Read the model definition and answer for the solid it produces. Units are mm, in the model's axes. Give positions to 0.01 mm unless a question says otherwise; leave off trailing zeros. Order: outer loops, then holes, each group sorted by start corner. A loop starts at its lowest first (then second) coordinate and runs counter-clockwise, first axis right, second up. Notation, with made-up numbers: (-35, 66) - (-27, 66) arc R23 ccw to (-27, 90) - close; hole circle Ø9 at (-23, -22.5). An arc over 180 degrees is marked (long way). Write item = value, one per line.
```python
from build123d import *

# Parameters (mm, degrees)
SKETCH1_R           = 46.575911091
SKETCH1_R_2         = 1.5875
BOSS_EXTRUDE1_DEPTH = 3.175


with BuildPart() as part:
    # Sketch1 → Boss-Extrude1 (new body)
    with BuildSketch(Plane(origin=(0, 0, 0), x_dir=(1, 0, 0), z_dir=(0, 1, 0))):
        with Locations(Location((-1e-09, -8.701819906, 0), (0, 0, 270))):
            Circle(SKETCH1_R)
        with Locations(Location((-21.062340002, 28.785905516, 0), (0, 0, 270))):
            Circle(SKETCH1_R_2, mode=Mode.SUBTRACT)
        with Locations(Location((20.847659998, 28.785905516, 0), (0, 0, 270))):
            Circle(SKETCH1_R_2, mode=Mode.SUBTRACT)
        with BuildLine():
            Line((17.640592508, -35.322668494), (1.122532008, -18.804607993))
            ThreePointArc((1.122532008, -18.804607993), (-8e-09, -18.339640008), (-1.122532023, -18.804607993))
            Line((-1.122532023, -18.804607993), (-17.640592542, -35.322668513))
            ThreePointArc((-17.640592542, -35.322668513), (-18.093334403, -36.641843516), (-17.330191572, -37.809238437))
            ThreePointArc((-17.330191572, -37.809238437), (-1.3e-08, -42.577730996), (17.330191539, -37.809238417))
            ThreePointArc((17.330191539, -37.809238417), (18.09333437, -36.641843496), (17.640592508, -35.322668494))
        make_face(mode=Mode.SUBTRACT)
        Polygon((-18.9752812, 8.136160364), (-16.837980243, 10.27346132), (-7.965487196, 1.400968273), (-10.102788153, -0.736332684), align=None, mode=Mode.SUBTRACT)
        with BuildLine():
            Line((26.620848619, -26.342412348), (10.102788136, -9.824351865))
            ThreePointArc((10.102788136, -9.824351865), (9.637820151, -8.70181985), (10.102788136, -7.579287835))
            Line((10.102788136, -7.579287835), (26.620848586, 8.938772615))
            ThreePointArc((26.620848586, 8.938772615), (27.940023589, 9.391514476), (29.107418509, 8.628371644))
            ThreePointArc((29.107418509, 8.628371644), (33.875911069, -8.70181986), (29.107418545, -26.032011374))
            ThreePointArc((29.107418545, -26.032011374), (27.940023624, -26.795154209), (26.620848619, -26.342412348))
        make_face(mode=Mode.SUBTRACT)
        with BuildLine():
            Line((-26.620848661, -26.342412387), (-10.102788145, -9.824351871))
            ThreePointArc((-10.102788145, -9.824351871), (-9.63782016, -8.701819856), (-10.102788145, -7.579287841))
            Line((-10.102788145, -7.579287841), (-26.620848632, 8.938772647))
            ThreePointArc((-26.620848632, 8.938772647), (-27.940023635, 9.391514508), (-29.107418555, 8.628371678))
            ThreePointArc((-29.107418555, 8.628371678), (-33.875911135, -8.701819865), (-29.107418586, -26.032011416))
            ThreePointArc((-29.107418586, -26.032011416), (-27.940023665, -26.795154248), (-26.620848661, -26.342412387))
        make_face(mode=Mode.SUBTRACT)
        Polygon((-18.975281171, -25.539800119), (-10.102788124, -16.667307072), (-7.965487167, -18.804608029), (-16.837980215, -27.677101076), align=None, mode=Mode.SUBTRACT)
        Polygon((-5.504897018, -12.069415894), (3.367596037, -3.196922839), (5.504896994, -5.334223796), (-3.367596061, -14.206716851), align=None, mode=Mode.SUBTRACT)
        Polygon((7.965487156, 1.40096828), (16.837980204, 10.273461327), (18.975281161, 8.13616037), (10.102788113, -0.736332677), align=None, mode=Mode.SUBTRACT)
        Polygon((7.965487164, -18.804608029), (10.102788121, -16.667307072), (18.975281169, -25.539800119), (16.837980212, -27.677101076), align=None, mode=Mode.SUBTRACT)
        with BuildLine():
            Line((-1.122532017, 1.400968288), (-17.640592486, 17.919028757))
            ThreePointArc((-17.640592486, 17.919028757), (-18.093334347, 19.238203762), (-17.330191513, 20.405598683))
            ThreePointArc((-17.330191513, 20.405598683), (-9e-09, 25.174091207), (17.330191488, 20.405598658))
            ThreePointArc((17.330191488, 20.405598658), (18.093334321, 19.238203738), (17.64059246, 17.919028734))
            Line((17.64059246, 17.919028734), (1.122532014, 1.400968288))
            ThreePointArc((1.122532014, 1.400968288), (-1e-09, 0.936000303), (-1.122532017, 1.400968288))
        make_face(mode=Mode.SUBTRACT)
        with BuildLine():
            ThreePointArc((-29.762524278, -33.966511802), (-29.579626476, -31.728910208), (-27.342024882, -31.911808011))
            ThreePointArc((-27.342024882, -31.911808011), (-25.360302369, -34.062122274), (-23.209988106, -36.043844786))
            ThreePointArc((-23.209988106, -36.043844786), (-23.027090304, -38.28144638), (-25.264691898, -38.464344183))
            ThreePointArc((-25.264691898, -38.464344183), (-27.605366399, -36.307186304), (-29.762524278, -33.966511802))
        make_face(mode=Mode.SUBTRACT)
        with BuildLine():
            ThreePointArc((23.000626318, -36.039350311), (22.807915825, -38.276128165), (25.044693679, -38.468838657))
            ThreePointArc((25.044693679, -38.468838657), (27.507381615, -36.209201522), (29.767018749, -33.746513584))
            ThreePointArc((29.767018749, -33.746513584), (29.574308255, -31.509735732), (27.337530403, -31.702446226))
            ThreePointArc((27.337530403, -31.702446226), (25.262317586, -33.964137493), (23.000626318, -36.039350311))
        make_face(mode=Mode.SUBTRACT)
    extrude(amount=BOSS_EXTRUDE1_DEPTH)


solid = part.part
```
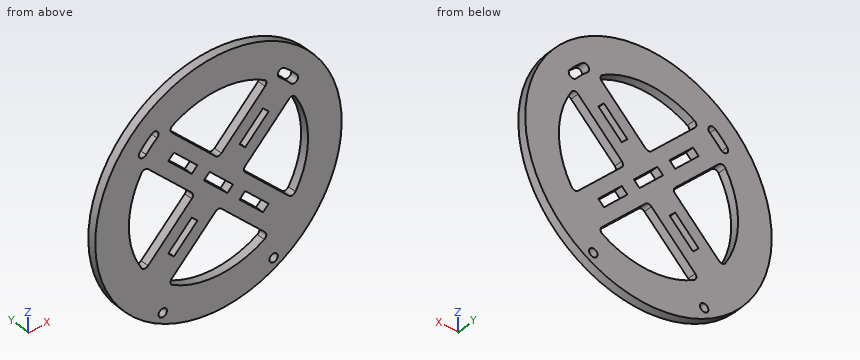
1. Straight lines are drawn through the part: L1, parallel to Z at x = -24, y = 1.35; L2, parallel to Z at x = 29, y = 3.05; L3, parallel to X at y = 2.6, z = 20. For each, find the intervals that lie inside material, in ascending order. Write a range as [from, to].
Recorded:
L1 = [-31.21, -6.32], [23.72, 35.35], [38.82, 48.62]
L2 = [-27.74, -8.79], [26.19, 31.2], [34.63, 45.15]
L3 = [-45.18, -31.94], [-20.28, -13.44], [-9.16, -2.32], [2.32, 9.16], [13.44, 20.28], [31.94, 45.18]
2. Section A-A (z = -16.5) is taken. Determine the outline of the cut face in (x, y) (3 decimals), and give its area (3 significant figures).
Recorded:
outline = (-39.169, 0) - (-16.222, 0) - (-16.222, 3.175) - (-39.169, 3.175) - close; (16.222, 0) - (39.169, 0) - (39.169, 3.175) - (16.222, 3.175) - close
area = 146 mm^2
3. Flat-ended cylindrical pins translate along their axes: pin 1 (2.5 mm diameter, centred on x = 20.85, z = -28.79, fed in from +Y); pin 2 (1 mm diameter, centred on y = 2, z = 10, fed in from -X). Find the tip coordinate at first contact, or state that the pin passes through.
Recorded:
pin_1 = through
pin_2 = -46.57
4. Section B-B (x = 0) is taken. Determine the outline of the cut face in (y, z) (3 decimals).
Recorded:
outline = (0, -37.874) - (3.175, -37.874) - (3.175, -25.174) - (0, -25.174) - close; (0, -0.936) - (3.175, -0.936) - (3.175, 6.565) - (0, 6.565) - close; (0, 10.839) - (3.175, 10.839) - (3.175, 18.34) - (0, 18.34) - close; (0, 42.578) - (3.175, 42.578) - (3.175, 55.278) - (0, 55.278) - close
5. Section C-C (y = 0.95) is taken. Count the separate pieces of the cut face and the enclosed holes in it, and give its area (3 significant figures).
Recorded:
separate_pieces = 1
enclosed_holes = 13
area = 4,510 mm^2
